Verification items for this drawing (mm, ordinates from the low corner). A direction names the side the tool comes from. Give positions to 0.01 mm unless a question says otherwise; leave off trailing zeros. Order: outer loops, then holes, each group sorted by start corner. A loop starts at its lowest first (then second) coordinate and runs counter-clockwise, first axis right, second up.
(1) Sectioned sample at D-D on z = 4.5. Record the cut outline in (x, y).
(2) Mould release check, pull along X, two halves, no side actions. Record for the marked faces 1, 2, 3 and 4: pulls with the +X half, pulls with the -X half, needs draft (parallel to the pull), parting line crosses it, or undercut.
(3) Sectioned sample at B-B on x = 16.75. Record the cut outline in (y, z), plus the area to 3 significant figures.
(4) Access from +Z, -Z, +X, -X, +Y, -Y to the whole of each face (thin tool, end or side, straight path). Record for the marked faces 5 and 6.
(5) Scan lines: L1, parallel to Y at x = 2.5, z = 3.7; L2, parallel to X at y = 3.3, z = 4.15; L3, parallel to X at y = 3.9, z = 2.45. Record each from-to range of solid material in increasing order.
(6) Sectioned sample at A-A on y = 2.47. Record the cut outline in (x, z).
(7) Sectioned sample at C-C on y = 0.8. Record the cut outline in (x, z), plus the area to 3 significant figures.
(8) Gauge pin test, flat ends, axial feed: pin 1 (2 mm diameter, centred on x = 6, z = 4, fed in from -Y); pin 2 (2 mm diameter, centred on x = 2.5, y = 2.47, fed in from -Z). Record the tip position at first contact, or that the pin passes through.
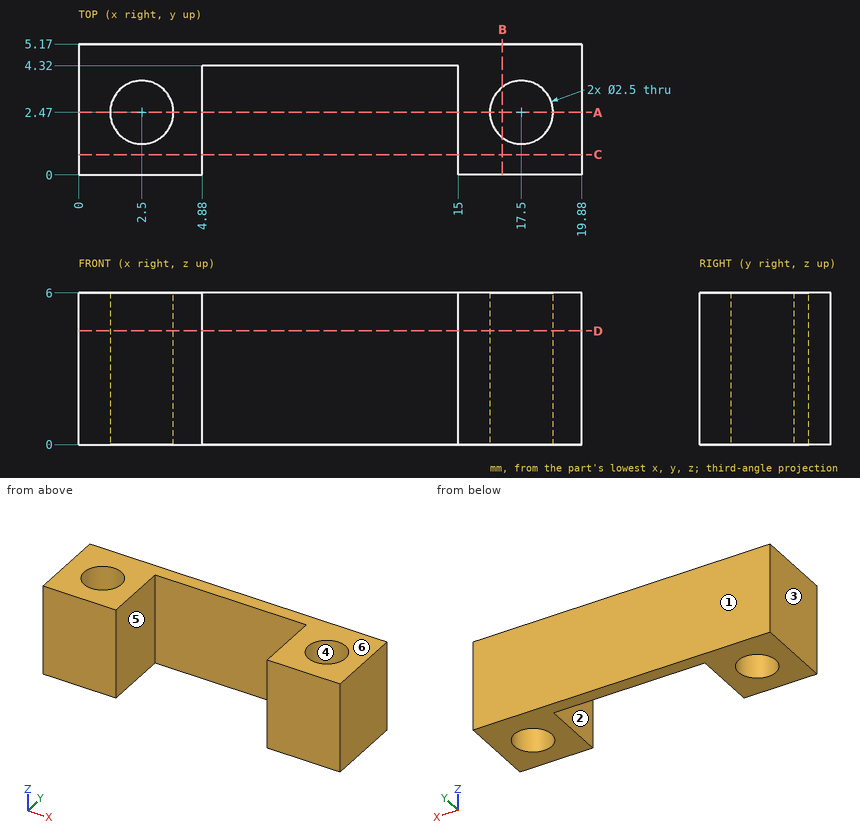
Ans:
1. outline: (0, 0) - (4.88, 0) - (4.88, 4.32) - (15, 4.32) - (15, 0) - (19.88, 0) - (19.88, 5.17) - (0, 5.17) - close; hole circle Ø2.5 at (2.5, 2.47); hole circle Ø2.5 at (17.5, 2.47)
2. face 1: needs draft
2. face 2: undercut
2. face 3: pulls with the -X half
2. face 4: undercut
3. outline: (0, 0) - (1.47, 0) - (1.47, 6) - (0, 6) - close; (3.47, 0) - (5.17, 0) - (5.17, 6) - (3.47, 6) - close
3. area: 19.0 mm2
4. face 5: +Z, -Z, -Y
4. face 6: +Z, +X, -X, +Y, -Y
5. L1: y = 0 to 1.22, 3.72 to 5.17
5. L2: x = 0 to 1.57, 3.43 to 4.88, 15 to 16.57, 18.43 to 19.88
5. L3: x = 0 to 4.88, 15 to 19.88
6. outline: (0, 0) - (1.25, 0) - (1.25, 6) - (0, 6) - close; (3.75, 0) - (4.88, 0) - (4.88, 6) - (3.75, 6) - close; (15, 0) - (16.25, 0) - (16.25, 6) - (15, 6) - close; (18.75, 0) - (19.88, 0) - (19.88, 6) - (18.75, 6) - close
7. outline: (0, 0) - (4.88, 0) - (4.88, 6) - (0, 6) - close; (15, 0) - (19.88, 0) - (19.88, 6) - (15, 6) - close
7. area: 58.6 mm2
8. pin 1: stops at y = 4.32
8. pin 2: passes through
